CAD build for the part. Positions are in the model's coordinates, mm. Face numbers are marked on the shaded views. A direction names the side the tool comes from. Give positions to 0.01 mm unless a question says otherwise; leave off trailing zeros. Order: outer loops, then holes, each group sorted by start corner. A loop starts at its lowest first (then second) coordinate and runs counter-clockwise, first axis right, second up.
Item 1: Wall check: L1, parallel to X at y = 59, z = 44; L2, parallel to Y at x = 5.5, z = 55; L3, parallel to X at y = 71, z = 9. Give the ranges that are in metal, low to high.
Item 2: Which spindle directions (+Z, -Z, +X, -X, +Y, -Y) get a long thin tool onto all of the face, cutting with end or side? Do the marked faces 5, 6 and 7. Say none if no direction does.
Item 3: Flat gauge pins, fed straight in: P1, Ø5, axis at x = 38, y = 58, coming from the +Z side; P2, Ø7.5, axis at x = 111, z = 74.5, coming from the +Y side; P3, Ø20.5, axis at x = -50.5, z = 50.5, coming from the +Y side; P4, Ø2, axis at x = 19, y = 62, coming from the +Z side. Where does each tip first touch, or does it go through?
Item 4: Two-plate mould, pull along Z, no slides. Class the marked faces 1, 2, 3 and 4: released by +Z, released by -Z, zero draft, split by the parting line, or undercut.
Item 5: Band-saw the part on A-A on y = 74. Give the cut face in (x, z), plus the area to 3 significant figures.
```python
from build123d import *

# Parameters (mm, degrees)
SKETCH1_W           = 203.2
SKETCH1_H           = 50.8
BOSS_EXTRUDE1_DEPTH = 88.9
SKETCH2_R           = 12.7
SKETCH2_R_2         = 25.4
CUT_EXTRUDE1_DEPTH  = 38.1
SKETCH3_R           = 12.7
CUT_EXTRUDE2_DEPTH  = 155.90300195
CUT_EXTRUDE3_DEPTH  = 30.48
FILLET1_R           = 2.54


with BuildPart() as part:
    # Sketch1 → Boss-Extrude1 (new body)
    with BuildSketch(Plane.XY):
        with Locations((19.396363636, 58.871863724)):
            Rectangle(SKETCH1_W, SKETCH1_H)
    extrude(amount=BOSS_EXTRUDE1_DEPTH)

    # Sketch2 → Cut-Extrude1 (cut)
    with BuildSketch(Plane(origin=(0, 84.271863724, 0), x_dir=(1, 0, 0), z_dir=(0, 1, 0))):
        with Locations(Location((-50.453636364, -44.45, 0), (0, 0, 180))):
            Circle(SKETCH2_R)
        with Locations((19.396363636, -88.9)):
            Circle(SKETCH2_R_2)
        with Locations((120.996363636, -88.9)):
            Circle(SKETCH2_R_2)
    extrude(amount=-CUT_EXTRUDE1_DEPTH, mode=Mode.SUBTRACT)

    # Sketch3 → Cut-Extrude2 (cut, through all)
    with BuildSketch(Plane(origin=(0, 46.171863724, 0), x_dir=(1, 0, 0), z_dir=(0, 1, 0))):
        with Locations((19.396363636, -88.9)):
            Circle(SKETCH3_R)
    extrude(amount=-CUT_EXTRUDE2_DEPTH, mode=Mode.SUBTRACT)

    # Sketch4 → Cut-Extrude3 (cut)
    with BuildSketch(Plane(origin=(0, 84.271863724, 0), x_dir=(1, 0, 0), z_dir=(0, 1, 0))):
        Polygon((-69.503636364, -88.9), (84.475680429, 0), (109.875680429, 0), (-44.103636364, -88.9), align=None)
    extrude(amount=-CUT_EXTRUDE3_DEPTH, mode=Mode.SUBTRACT)

    # Fillet1
    fillet1_edges = [part.edges().sort_by_distance(p)[0] for p in [
        (7.486022033, 53.791863724, 44.45),
        (32.886022033, 53.791863724, 44.45),
    ]]
    fillet(fillet1_edges, radius=FILLET1_R)


solid = part.part
```
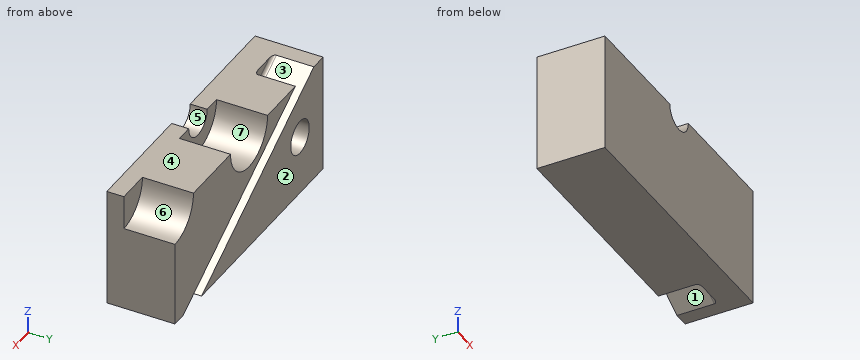
The answers:
1. L1: x = -82.2 to -63.15, -37.76 to 8.27, 33.67 to 121
1. L2: y = 33.47 to 53.79
1. L3: x = -82.2 to 68.89, 94.29 to 121
2. face 5: +Z, +Y, -Y
2. face 6: +Z, +X, +Y
2. face 7: +Z, +Y
3. P1: stops at z = 74.77
3. P2: stops at y = 46.17
3. P3: stops at y = 84.27
3. P4: stops at z = 63.54
4. face 1: undercut
4. face 2: zero draft
4. face 3: undercut
4. face 4: released by +Z
5. outline: (-82.2, 0) - (84.48, 0) - (-69.5, 88.9) - (-82.2, 88.9) - close; (-44.1, 88.9) - (109.88, 0) - (121, 0) - (121, 63.5) arc R25.4 cw to (95.6, 88.9) - (44.8, 88.9) arc R25.4 cw to (-6, 88.9) - close; hole circle Ø25.4 at (-50.45, 44.45)
5. area: 13,800 mm2
